from build123d import *

# Parameters (mm, degrees)
F0_R     = 10.070149
F1_DEPTH = 25.4
F2_DEPTH = 30.48


with BuildPart() as f1:
    # F0 (on Right) → F1 (new body)
    with BuildSketch(Plane.YZ):
        with BuildLine():
            ThreePointArc((-29.356436, 0), (0, -29.356436), (29.356436, 0))
            ThreePointArc((29.356436, 0), (0, 29.356436), (-29.356436, 0))
        make_face()
        Circle(F0_R, mode=Mode.SUBTRACT)
        with BuildLine():
            ThreePointArc((-29.356436, 0), (0, 29.356436), (29.356436, 0))
            Line((29.356436, 0), (29.356436, 71.070336))
            ThreePointArc((29.356436, 71.070336), (29.354923, 71.368341), (29.350386, 71.666315))
            ThreePointArc((29.350386, 71.666315), (0, 100.426772), (-29.350386, 71.666315))
            ThreePointArc((-29.350386, 71.666315), (-29.354923, 71.368341), (-29.356436, 71.070336))
            Line((-29.356436, 71.070336), (-29.356436, 0))
        make_face()
        with Locations((0, 71.666315)):
            Circle(F0_R, mode=Mode.SUBTRACT)
        with BuildLine():
            ThreePointArc((29.350386, 71.666315), (29.354923, 71.368341), (29.356436, 71.070336))
            Line((29.356436, 71.070336), (29.356436, 71.666315))
            Line((29.356436, 71.666315), (29.350386, 71.666315))
        make_face()
        with BuildLine():
            Line((-29.356436, 71.666315), (-29.356436, 71.070336))
            ThreePointArc((-29.356436, 71.070336), (-29.354923, 71.368341), (-29.350386, 71.666315))
            Line((-29.350386, 71.666315), (-29.356436, 71.666315))
        make_face()
    extrude(amount=F1_DEPTH)

    # F0 (on Right) → F2 (join)
    with BuildSketch(Plane.YZ):
        with BuildLine():
            ThreePointArc((-29.356436, 0), (0, -29.356436), (29.356436, 0))
            ThreePointArc((29.356436, 0), (0, 29.356436), (-29.356436, 0))
        make_face()
        Circle(F0_R, mode=Mode.SUBTRACT)
    extrude(amount=-F2_DEPTH)

    # F4: F1 across plane


with BuildPart() as f1_1:
    add(f1.part)
    add(f1.part.mirror(Plane(origin=(-30.48, 0, 0), x_dir=(0, 1, 0), z_dir=(-1, 0, 0))))


solid = f1_1.part
For this review, take the finished solid that the model builds, in its own axes (mm). Round coordinates to 2 decimals unless told otherwise and drop trailing zeros. Write each loop counter-clockwise with the first axis right and the second up, starting at its lowest first coordinate (ties: lowest second). Pieces come first, ordered by that corner, then holes. Notation, with made-up numbers: (-29.5, -19) -> (11.5, -19) arc R27 ccw to (11.5, 7) -> close; hole circle Ø2 at (14, 17.25). An arc over 180 degrees is marked (long way). Use CSV: the item, a comma, the result in double quotes.
(1) Draft analysis for pull direction Z (two halves, no side actions). For faces 1 (the face through (13, 29.356, 35)), 2 (the face through (12.52, -1.31, 81.65)), 3 (the face through (-73.48, 0.64, 100.42)), 4 (the face through (-73.48, -1.31, 81.65)), state which applies: +Z half, -Z half, draft (parallel to the pull), parting line (faces both ways), or undercut.
Computed values:
face 1,"draft"
face 2,"undercut"
face 3,"+Z half"
face 4,"undercut"
(2) Consider section C-C, the plane y = 0. Give the boundary of the cut face in (x, z).
Computed values:
outline,"(-86.36, -29.36) -> (25.4, -29.36) -> (25.4, -10.07) -> (-86.36, -10.07) -> close; (-86.36, 10.07) -> (25.4, 10.07) -> (25.4, 61.6) -> (0, 61.6) -> (0, 29.36) -> (-60.96, 29.36) -> (-60.96, 61.6) -> (-86.36, 61.6) -> close; (-86.36, 81.74) -> (-60.96, 81.74) -> (-60.96, 100.43) -> (-86.36, 100.43) -> close; (0, 81.74) -> (25.4, 81.74) -> (25.4, 100.43) -> (0, 100.43) -> close"
(3) Clearance check with flat-ended pins moving along their axes: P1, Ø12, axis at x = -43.5, z = 32, coming from the -Y side; P2, Ø10, axis at x = -53, y = 13.5, coming from the -Z side; P3, Ø10, axis at x = -17.5, z = -6, coming from the -Y side. State where each tip first meets the part, or that it passes through.
Computed values:
P1,"y = -13.63"
P2,"z = -28.1"
P3,"y = -29.34"
(4) Consider section A-A, the plane z = 60. Give the boundary of the cut face in (x, y), plus the area to 3 significant figures.
Computed values:
outline,"(-86.36, -29.36) -> (-60.96, -29.36) -> (-60.96, 29.36) -> (-86.36, 29.36) -> close; (0, -29.36) -> (25.4, -29.36) -> (25.4, 29.36) -> (0, 29.36) -> close"
area,"2,980 mm²"
(5) To check wall thickness, follow L1, parallel to Z at x = -17, y = 0; L2, parallel to X at y = -19, z = 66; L3, parallel to Y at x = 10.5, z = 2. State the ranges of each line that lie inside material, in increasing order. Write a range as [from, to].
Computed values:
L1,"[-29.36, -10.07], [10.07, 29.36]"
L2,"[-86.36, -60.96], [0, 25.4]"
L3,"[-29.36, -9.87], [9.87, 29.36]"
(6) Consider section B-B, the plane x = 3. Give the number of separate pieces and of enclosed holes in the cut face, plus the area to 3 significant figures.
Computed values:
separate pieces,"1"
enclosed holes,"2"
area,"6,240 mm²"
(7) Consider section D-D, the plane x = -42. Give the boundary of the cut face in (y, z), plus the area to 3 significant figures.
Computed values:
outline,"circle Ø58.71 at (0, 0); hole circle Ø20.14 at (0, 0)"
area,"2,390 mm²"
